from build123d import *

# Parameters (mm, degrees)
F0_W           = 20
F0_H           = 18
F1_DEPTH       = 2
F2_W           = 20
F2_H           = 1.9
F3_DEPTH       = 10
F4_W           = 20
F4_H           = 1.9
F5_DEPTH       = 1.9
F6_W           = 20
F6_H           = 1.9
F7_DEPTH       = 1.9
F8_R           = 4.5
F8_R_2         = 2
F9_DEPTH       = 4
F10_DEPTH      = 25
F11_W          = 8
F11_H          = 8.1
F11_H_2        = 4.5868207008
F12_DEPTH      = 19.901
F12_DEPTH_BACK = 25


with BuildPart() as f1:
    # F0 (on Top) → F1 (new body)
    with BuildSketch(Plane.XY):
        with Locations((-10, 9)):
            Rectangle(F0_W, F0_H)
    extrude(amount=F1_DEPTH)

    # F2 (on face) → F3 (join)
    with BuildSketch(Plane(origin=(0, 0, 0), x_dir=(1, 0, 0), z_dir=(0, 0, -1))):
        with Locations((-10, -0.95)):
            Rectangle(F2_W, F2_H)
        with Locations((-10, -17.05)):
            Rectangle(F2_W, F2_H)
    extrude(amount=F3_DEPTH)

    # F4 (on face) → F5 (join)
    with BuildSketch(Plane.XZ):
        with Locations((-10, -9.05)):
            Rectangle(F4_W, F4_H)
    extrude(amount=F5_DEPTH)

    # F6 (on face) → F7 (join)
    with BuildSketch(Plane(origin=(0, 18, 0), x_dir=(-1, 0, 0), z_dir=(0, 1, 0))):
        with Locations((10, -9.05)):
            Rectangle(F6_W, F6_H)
    extrude(amount=F7_DEPTH)

    # F8 (on face) → F9 (join)
    with BuildSketch(Plane.XY.offset(2)):
        with Locations((-10, 9)):
            Circle(F8_R)
        with Locations((-10, 9)):
            Circle(F8_R_2, mode=Mode.SUBTRACT)
    extrude(amount=F9_DEPTH)

    # F10 (add): a face of the model
    f10_faces = [f1.faces().sort_by_distance(p)[0] for p in [
        (-10, 9, 2),
    ]]
    extrude(f10_faces, amount=F10_DEPTH)

    # F11 (on face) → F12 (cut, two sides)
    with BuildSketch(Plane.XZ) as f12_sk:
        with Locations((-10, -4.05)):
            Rectangle(F11_W, F11_H)
        with Locations((-10, -10.3934103504)):
            Rectangle(F11_W, F11_H_2)
    extrude(amount=-F12_DEPTH, mode=Mode.SUBTRACT)
    extrude(f12_sk.sketch, amount=F12_DEPTH_BACK, mode=Mode.SUBTRACT)


solid = f1.part
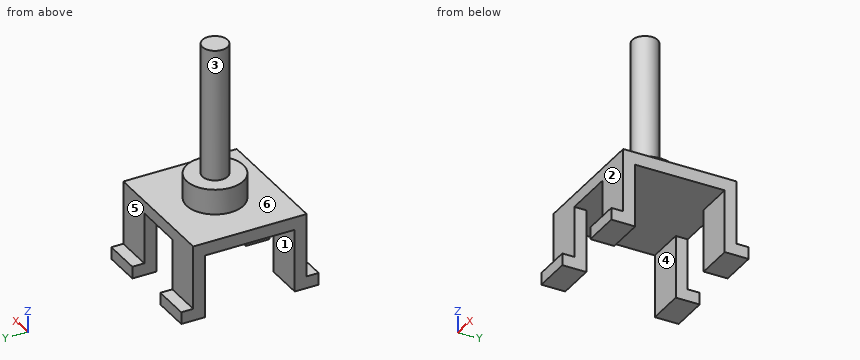
Part model, mm, in its own coordinate system. Face numbers are marked on the shaded views. A direction names the side the tool comes from. Round coordinates to 2 decimals unless told otherwise and drop trailing zeros. Write each loop counter-clockwise with the first axis right and the second up, starting at its lowest first coordinate (ties: lowest second). Pieces come first, ordered by that corner, then holes. Notation, with made-up numbers: M 34.5,-26.5 L 79.5,-26.5 A21 ccw 79.5,-8.5 Z; hole C 56.5,5 d3. An arc over 180 degrees is marked long. Return JSON: item names as keys, results as strings. Group by question number.
(1) Saw through at B-B on x = -10. Write the cut outline in (y, z), then the cut area to 3 significant figures.
(2) Drill centre lines: probe 1 along Y at (x, z) = (-14.25, -4); probe 2 along X at (y, z) = (17.5, -5); probe 3 along Z at (x, y) = (-4, 15). Where is each one in solid material? Low to high.
(3) Two-plate mould, pull along Y, no slides. Class the marked faces 1, 2 and 3: +Y half, -Y half, draft (parallel to the pull), parting line (faces both ways), or undercut.
(4) Saw through at D-D on z = 18. Write the cut outline in (x, y), then the cut area to 3 significant figures.
(5) Saw through at C-C on y = 9. Write the cut outline in (x, z).
(6) Saw through at A-A on z = -3. Write the cut outline in (x, y).
(7) Which spindle directions (+Z, -Z, +X, -X, +Y, -Y) get a long thin tool onto all of the face, cutting with end or side? Do the marked faces 4, 5 and 6. Say none if no direction does.
(8) Pin check, flat tips, straight feed: pin 1 Ø3 at (x, y) = (-16, 4.5) entering from -Z; pin 2 Ø1 at (x, z) = (-8.5, 2) entering from +Y; pin 3 Ø1.5 at (x, y) = (-16, 19.5) entering from +Z. Stop position of each tip, or through.
Returned:
{
 "1": {"outline": "M 0,0 L 18,0 L 18,2 L 13.5,2 L 13.5,6 L 11,6 L 11,27 L 7,27 L 7,6 L 4.5,6 L 4.5,2 L 0,2 Z", "area": "156 mm²"},
 "2": {"probe 1": "0 to 1.9, 16.1 to 18", "probe 2": "-20 to -14, -6 to 0", "probe 3": "0 to 2"},
 "3": {"face 1": "undercut", "face 2": "-Y half", "face 3": "parting line"},
 "4": {"outline": "C -10,9 d4", "area": "12.6 mm²"},
 "5": {"outline": "M -20,0 L 0,0 L 0,2 L -5.5,2 L -5.5,6 L -8,6 L -8,27 L -12,27 L -12,6 L -14.5,6 L -14.5,2 L -20,2 Z"},
 "6": {"outline": "M -20,0 L -14,0 L -14,1.9 L -20,1.9 Z; M -20,16.1 L -14,16.1 L -14,18 L -20,18 Z; M -6,0 L 0,0 L 0,1.9 L -6,1.9 Z; M -6,16.1 L 0,16.1 L 0,18 L -6,18 Z"},
 "7": {"face 4": "-Z, +X, -X", "face 5": "+Z, +X, -X, +Y", "face 6": "+Z"},
 "8": {"pin 1": "z = 0", "pin 2": "y = 18", "pin 3": "z = -8.1"}
}
